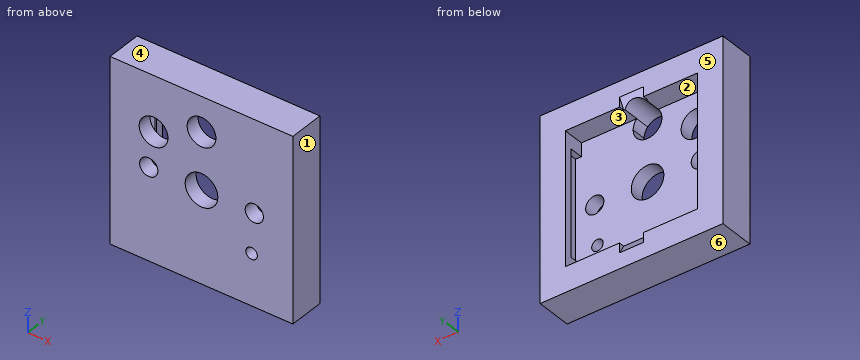
from build123d import *

# Parameters (mm, degrees)
SKETCH1_W           = 19.05
SKETCH1_H           = 19.05
SKETCH1_R           = 1.5
SKETCH1_R_2         = 0.95
SKETCH1_R_3         = 1.7
SKETCH1_R_4         = 0.6
BOSS_EXTRUDE1_DEPTH = 3.7
CUT_EXTRUDE1_START  = 3.7
SKETCH1_3_R         = 1.5
SKETCH1_3_R_2       = 0.95
SKETCH1_3_R_3       = 1.7
SKETCH1_3_R_4       = 0.6
CUT_EXTRUDE1_DEPTH  = 2.2
CUT_EXTRUDE2_DEPTH  = 1.25
CUT_EXTRUDE3_DEPTH  = 5.5


with BuildPart() as part:
    # Sketch1 → Boss-Extrude1 (new body)
    with BuildSketch(Plane(origin=(0, 0, 0), x_dir=(1, 0, 0), z_dir=(0, 1, 0))):
        Rectangle(SKETCH1_W, SKETCH1_H)
        with BuildLine():
            Line((-6.9, -6.9), (-6.9, 6.9))
            Line((-6.9, 6.9), (6.9, 6.9))
            Line((6.9, 6.9), (6.9, -6.9))
            Line((6.9, -6.9), (1.118033989, -6.9))
            ThreePointArc((1.118033989, -6.9), (0, -7.4), (-1.118033989, -6.9))
            Line((-1.118033989, -6.9), (-6.9, -6.9))
        make_face(mode=Mode.SUBTRACT)
        with BuildLine():
            Line((6.9, 6.9), (-6.9, 6.9))
            Line((-6.9, 6.9), (-6.9, -6.9))
            Line((-6.9, -6.9), (-1.118033989, -6.9))
            ThreePointArc((-1.118033989, -6.9), (-0.535233135, -4.498741462), (1.5, -5.9))
            ThreePointArc((1.5, -5.9), (1.401258538, -6.435233135), (1.118033989, -6.9))
            Line((1.118033989, -6.9), (6.9, -6.9))
            Line((6.9, -6.9), (6.9, 6.9))
        make_face()
        with Locations((-5, -3.8)):
            Circle(SKETCH1_R, mode=Mode.SUBTRACT)
        with Locations((5.5, 0)):
            Circle(SKETCH1_R_2, mode=Mode.SUBTRACT)
        with Locations((-5.5, 0)):
            Circle(SKETCH1_R_2, mode=Mode.SUBTRACT)
        Circle(SKETCH1_R_3, mode=Mode.SUBTRACT)
        with Locations((5.22, 4.2)):
            Circle(SKETCH1_R_4, mode=Mode.SUBTRACT)
    extrude(amount=BOSS_EXTRUDE1_DEPTH)

    # Sketch1<3> → Cut-Extrude1 (cut)
    with BuildSketch(Plane(origin=(0, 0, 0), x_dir=(1, 0, 0), z_dir=(0, 1, 0)).offset(CUT_EXTRUDE1_START)):
        with BuildLine():
            Line((6.9, 6.9), (-6.9, 6.9))
            Line((-6.9, 6.9), (-6.9, -6.9))
            Line((-6.9, -6.9), (-1.118033989, -6.9))
            ThreePointArc((-1.118033989, -6.9), (-0.535233135, -4.498741462), (1.5, -5.9))
            ThreePointArc((1.5, -5.9), (1.401258538, -6.435233135), (1.118033989, -6.9))
            Line((1.118033989, -6.9), (6.9, -6.9))
            Line((6.9, -6.9), (6.9, 6.9))
        make_face()
        with Locations((-5, -3.8)):
            Circle(SKETCH1_3_R, mode=Mode.SUBTRACT)
        with Locations((5.5, 0)):
            Circle(SKETCH1_3_R_2, mode=Mode.SUBTRACT)
        with Locations((-5.5, 0)):
            Circle(SKETCH1_3_R_2, mode=Mode.SUBTRACT)
        Circle(SKETCH1_3_R_3, mode=Mode.SUBTRACT)
        with Locations((5.22, 4.2)):
            Circle(SKETCH1_3_R_4, mode=Mode.SUBTRACT)
    extrude(amount=-CUT_EXTRUDE1_DEPTH, mode=Mode.SUBTRACT)

    # Sketch2 → Cut-Extrude2 (cut, symmetric)
    with BuildSketch(Plane(origin=(0, 0, 0), x_dir=(0, 0, -1), z_dir=(1, 0, 0))):
        Polygon((-7.9, 3.7), (-6.9, 3.7), (-6.9, 3.122649731), align=None)
    cut_extrude2 = extrude(amount=CUT_EXTRUDE2_DEPTH, both=True, mode=Mode.SUBTRACT)

    # Mirror1: Cut-Extrude2 across plane
    add(cut_extrude2.mirror(Plane.XY), mode=Mode.SUBTRACT)

    # Sketch4 → Cut-Extrude3 (cut, symmetric)
    with BuildSketch(Plane.XY):
        Polygon((-6.9, 2.9), (-6.9, 1.5), (-7.5, 1.5), (-7.5, 2.8), (-7, 2.8), align=None)
    cut_extrude3 = extrude(amount=CUT_EXTRUDE3_DEPTH, both=True, mode=Mode.SUBTRACT)

    # Mirror2: Cut-Extrude3 across plane
    add(cut_extrude3.mirror(Plane(origin=(0, 0, 0), x_dir=(0, 0, 1), z_dir=(1, 0, 0))), mode=Mode.SUBTRACT)


solid = part.part
CAD build for the part. Positions are in the model's coordinates, mm. Face numbers are marked on the shaded views. A direction names the side the tool comes from. Coordinates: 2 decimals unless noted, no trailing zeros. Write each loop counter-clockwise with the first axis right and the second up, starting at its lowest first coordinate (ties: lowest second). Pieces come first, ordered by that corner, then holes. Notation, with made-up numbers: M -32,-4.5 L 23,-4.5 A29 ccw 23,24.5 Z; hole C 28.25,55.25 d11. An arc over 180 degrees is marked long. Return JSON: item names as keys, results as strings.
Item 1: Two-plate mould, pull along Z, no slides. Class the marked faces 3, 4, 5 and 6: +Z half, -Z half, draft (parallel to the pull), parting line (faces both ways), or undercut.
Findings below:
{"face 3": "undercut", "face 4": "+Z half", "face 5": "draft", "face 6": "-Z half"}
Item 2: Probe line 1 (X direction, y = 0.4, z = 0) (3 decimals); line 2 (Z direction, x = -3, y = 1.85) (3 decimals); line 3 (Z direction, x = 0, y = 1.25) (3 decimals). List the from-to ranges inside material, lowest first. Write a range as from..to.
Findings below:
{"line 1": "x = -9.525..-6.45, -4.55..-1.7, 1.7..4.55, 6.45..9.525", "line 2": "z = -9.525..-6.9, 6.9..9.525", "line 3": "z = -9.525..-1.7, 1.7..4.4, 7.4..9.525"}
Item 3: Slice it at B-B, the plane z = -4.2. Write the cut outline in (x, y) (3 decimals), and give its area (3 significant figures).
Findings below:
{"outline": "M -9.525,0 L 4.62,0 L 4.62,1.5 L -7.5,1.5 L -7.5,2.8 L -7,2.8 L -6.9,2.9 L -6.9,3.7 L -9.525,3.7 Z; M 5.82,0 L 9.525,0 L 9.525,3.7 L 6.9,3.7 L 6.9,2.9 L 7,2.8 L 7.5,2.8 L 7.5,1.5 L 5.82,1.5 Z", "area": "36.8 mm2"}
Item 4: Slice it at D-D, the plane z = 0. Write the cut outline in (x, y) (3 decimals).
Findings below:
{"outline": "M -9.525,0 L -6.45,0 L -6.45,1.5 L -7.5,1.5 L -7.5,2.8 L -7,2.8 L -6.9,2.9 L -6.9,3.7 L -9.525,3.7 Z; M -4.55,0 L -1.7,0 L -1.7,1.5 L -4.55,1.5 Z; M 1.7,0 L 4.55,0 L 4.55,1.5 L 1.7,1.5 Z; M 6.45,0 L 9.525,0 L 9.525,3.7 L 6.9,3.7 L 6.9,2.9 L 7,2.8 L 7.5,2.8 L 7.5,1.5 L 6.45,1.5 Z"}
Item 5: Slice it at A-A, the plane x = 0. Write the cut outline in (y, z) (3 decimals).
Findings below:
{"outline": "M 0,-9.525 L 3.7,-9.525 L 3.7,-7.9 L 3.123,-6.9 L 1.5,-6.9 L 1.5,-1.7 L 0,-1.7 Z; M 0,1.7 L 1.5,1.7 L 1.5,4.4 L 0,4.4 Z; M 0,7.4 L 3.411,7.4 L 3.7,7.9 L 3.7,9.525 L 0,9.525 Z"}
Item 6: Which spindle directions (+Z, -Z, +X, -X, +Y, -Y) get a long thin tool onto all of the face, cutting with end or side? Do the marked faces 1 and 2. Say none if no direction does.
Findings below:
{"face 1": "+Z, -Z, +X, +Y, -Y", "face 2": "+Y"}
Item 7: Slice it at C-C, the plane y = 2.25. Write the cut outline in (x, z) (3 decimals), and give its area (3 significant figures).
Findings below:
{"outline": "M -9.525,-9.525 L 9.525,-9.525 L 9.525,9.525 L -9.525,9.525 Z; hole M -7.5,-5.5 L -6.9,-5.5 L -6.9,-6.9 L 6.9,-6.9 L 6.9,-5.5 L 7.5,-5.5 L 7.5,5.5 L 6.9,5.5 L 6.9,6.9 L 1.118,6.9 A1.5 ccw -1.118,6.9 L -6.9,6.9 L -6.9,5.5 L -7.5,5.5 Z", "area": "158 mm2"}
